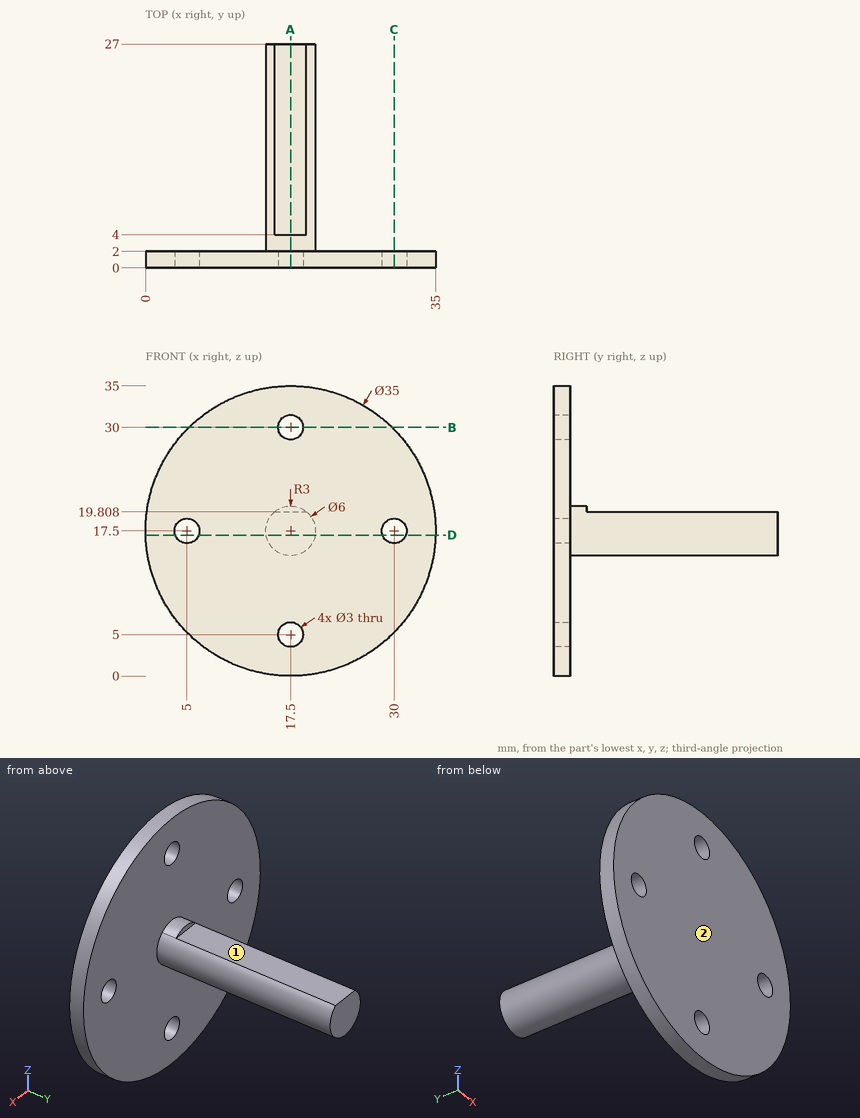
The drawing under review shows one solid part. Ordinate dimensions are in mm from its lowest x, y, z. A direction names the side the tool comes from. Coordinates: 2 decimals unless noted, no trailing zeros. Write each loop counter-clockwise with the first axis right and the second up, starting at its lowest first coordinate (ties: lowest second). Pieces come first, ordered by that corner, then holes. Notation, with made-up numbers: M 41,-22 L 54,-22 A11 ccw 54,-2 Z; hole C 17,-24 d4. An arc over 180 degrees is marked long. Put each result on its own line as item: value.
1) Wall thickness on probe 1 along X at (y, z) = (1.4, 17.5); probe 2 along X at (y, z) = (1.05, 30); probe 3 along Y at (x, z) = (26.5, 10.5): over which ranges is each line inside the solid? List them lowest first. Write a range as [from, to].
Computed:
probe 1: x = [0, 3.5], [6.5, 28.5], [31.5, 35]
probe 2: x = [5.25, 16], [19, 29.75]
probe 3: y = [0, 2]
2) For the marked faces 1 and 2, list the 3-axis set-ups (+Z, -Z, +X, -X, +Y, -Y) from which the entire face can be reached by the end or side of a thin tool; tool diameter is ignored.
Computed:
face 1: +Z, +X, -X, +Y
face 2: +Z, -Z, +X, -X, -Y
3) Clearance check with flat-ended pins moving along their axes: pin 1 Ø3 at (x, y) = (17.5, 16.5) entering from +Z; pin 2 Ø6 at (x, z) = (10, 13) entering from +Y; pin 3 Ø6 at (y, z) = (14.5, 22) entering from +X. State where each tip first meets the part, or that it passes through.
Computed:
pin 1: stops at z = 19.81
pin 2: stops at y = 2
pin 3: stops at x = 20.1
4) Add section A-A on x = 17.5. Give the boundary of the cut face in (y, z), then the cut area to 3 significant figures.
Computed:
outline: M 0,0 L 2,0 L 2,3.5 L 0,3.5 Z; M 0,6.5 L 2,6.5 L 2,14.5 L 27,14.5 L 27,19.81 L 4,19.81 L 4,20.5 L 2,20.5 L 2,28.5 L 0,28.5 Z; M 0,31.5 L 2,31.5 L 2,35 L 0,35 Z
area: 192 mm2
5) Add section C-C on x = 30. Give the boundary of the cut face in (y, z), then the cut area to 3 significant figures.
Computed:
outline: M 0,5.25 L 2,5.25 L 2,16 L 0,16 Z; M 0,19 L 2,19 L 2,29.75 L 0,29.75 Z
area: 43.0 mm2
6) Add section B-B on z = 30. Give the boundary of the cut face in (x, y), then the cut area to 3 significant figures.
Computed:
outline: M 5.25,0 L 16,0 L 16,2 L 5.25,2 Z; M 19,0 L 29.75,0 L 29.75,2 L 19,2 Z
area: 43.0 mm2
7) Add section D-D on z = 17. Give the boundary of the cut face in (x, y), then the cut area to 3 significant figures.
Computed:
outline: M 0.01,0 L 3.59,0 L 3.59,2 L 0.01,2 Z; M 6.41,0 L 28.59,0 L 28.59,2 L 20.46,2 L 20.46,27 L 14.54,27 L 14.54,2 L 6.41,2 Z; M 31.41,0 L 34.99,0 L 34.99,2 L 31.41,2 Z
area: 207 mm2
